Read the model definition and answer for the solid it produces. Units are mm, in the model's axes. Face numbers are marked on the shaded views. A direction names the side the tool comes from. Give positions to 0.01 mm unless a question says otherwise; leave off trailing zeros. Order: outer loops, then holes, each group sorted by start corner. A loop starts at its lowest first (then second) coordinate and runs counter-clockwise, first axis right, second up. Notation, with made-up numbers: M 85.25,66 L 132.25,66 A7 ccw 132.25,73 Z; hole C 72.5,-2.75 d4. An arc over 180 degrees is marked long. One line per item, written item: value. Start each with the question number.
Autodesk Inventor part; units mm, degrees
ref_plane "YZ Plane" through (0, 0, 0) normal (1, 0, 0) x (0, 1, 0)
ref_plane "XZ Plane" through (0, 0, 0) normal (0, 1, 0) x (-1, 0, 0)
ref_plane "XY Plane" through (0, 0, 0) normal (0, 0, 1) x (1, 0, 0)
sketch "スケッチ1" plane through (0, 0, 0) normal (0, 1, 0) x (-1, 0, 0)
  circle A0 centre (0, 0) radius 32.5
  dimension "d0" = 65
extrude "押し出し1" add sketch "スケッチ1" along normal blind 5.8
sketch "スケッチ2" plane through (0, 5.8, 0) normal (0, 1, 0) x (1, 0, 0)
  circle A0 centre (0, 0) radius 18
  dimension "d3" = 36
extrude "押し出し2" cut sketch "スケッチ2" against normal through all
sketch "スケッチ3" plane through (0, 0, 0) normal (0, -1, 0) x (1, 0, 0)
  circle A0 centre (0, 0) radius 25.15
  dimension "d6" = 50.3
extrude "押し出し3" cut sketch "スケッチ3" against normal blind 5.3
sketch "スケッチ4" plane through (0, 5.8, 0) normal (0, 1, 0) x (1, 0, 0)
  circle A0 centre (0, 0) radius 32.5
  circle A1 centre (0, 0) radius 25.65
  dimension "d9" = 51.3
extrude "押し出し4" cut sketch "スケッチ4" against normal blind 5.3
sketch "スケッチ5" plane through (0, 0.5, 0) normal (0, 1, 0) x (1, 0, 0)
  circle A0 centre (0, 29) radius 1.65
  circle A1 centre (-25.1147, -14.5) radius 1.65
  circle A2 centre (25.1147, -14.5) radius 1.65
  point P0 (0, 0)
  dimension "d12" = 3.3
  dimension "d13" = 29
  dimension "d16" = 360
extrude "押し出し5" cut sketch "スケッチ5" against normal through all
properties part number "clamp_for_bearing" material "ステンレス鋼"
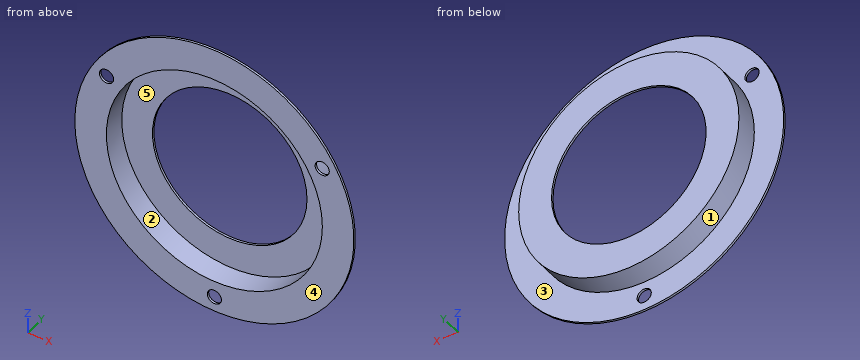
Q1. Find section C-C, the plane x = -17. Give the vertices of the cut face in (y, z), then the cut area to 3 significant figures.
Q2. Find section A-A, the plane x = 0. Give the vertices of the cut face in (y, z).
Q3. Determine the mould class of the marked faces 1, 2 and 3 for opening direction X: released by +X, released by -X, zero draft, split by the parting line, or undercut.
Q4. Consider probe 1 along X at (y, z) = (0.2, 14.5); probe 2 along X at (y, z) = (0.85, -0.5); probe 3 along X at (y, z) = (5.55, 0). Determine where each line is inside the solid, lowest interval first.
Q5. Find section B-B, the plane z = 0. Give the vertices of the cut face in (x, y).
Q6. A tool of negligible diameter and unlimited length cuts with its end or side. For the marked faces 4 and 5, from which of +Z, -Z, +X, -X, +Y, -Y can it reach the whole face along a straight path? Write none if from no direction.
Q7. Find section D-D, the plane z = 14.5. Give the vertices of the cut face in (x, y), then the cut area to 3 significant figures.
Q8. Each of these flat-tipped pins is pushed along its axis until it touches: pin 1 (4.5 mm diameter, centred on x = 25.11, z = 14.5, fed in from +Y); pin 2 (25 mm diameter, centred on x = -7, z = -5, fed in from -Y); pin 3 (1 mm diameter, centred on x = -13.5, y = 0.5, fed in from +Z). Where does it stop, or does it pass through?
Evaluation:
1. outline: M 0,-27.7 L 0.5,-27.7 L 0.5,-19.21 L 5.8,-19.21 L 5.8,-5.92 L 5.3,-5.92 L 5.3,-18.53 L 0,-18.53 Z; M 0,18.53 L 5.3,18.53 L 5.3,5.92 L 5.8,5.92 L 5.8,19.21 L 0.5,19.21 L 0.5,27.7 L 0,27.7 Z
1. area: 28.9 mm2
2. outline: M 0,-32.5 L 0.5,-32.5 L 0.5,-30.65 L 0,-30.65 Z; M 0,-27.35 L 0.5,-27.35 L 0.5,-25.65 L 5.8,-25.65 L 5.8,-18 L 5.3,-18 L 5.3,-25.15 L 0,-25.15 Z; M 0,25.15 L 5.3,25.15 L 5.3,18 L 5.8,18 L 5.8,25.65 L 0.5,25.65 L 0.5,32.5 L 0,32.5 Z
3. face 1: split by the parting line
3. face 2: undercut
3. face 3: zero draft
4. probe 1: -29.09 to -26.76, -23.46 to -20.55, 20.55 to 23.46, 26.76 to 29.09
4. probe 2: -25.65 to -25.15, 25.15 to 25.65
4. probe 3: -25.65 to -18, 18 to 25.65
5. outline: M -32.5,0 L -25.15,0 L -25.15,5.3 L -18,5.3 L -18,5.8 L -25.65,5.8 L -25.65,0.5 L -32.5,0.5 Z; M 18,5.3 L 25.15,5.3 L 25.15,0 L 32.5,0 L 32.5,0.5 L 25.65,0.5 L 25.65,5.8 L 18,5.8 Z
6. face 4: +Z, -Z, +X, -X, -Y
6. face 5: -Y
7. outline: M -29.09,0 L -26.76,0 L -26.76,0.5 L -29.09,0.5 Z; M -23.46,0 L -20.55,0 L -20.55,5.3 L -10.67,5.3 L -10.67,5.8 L -21.16,5.8 L -21.16,0.5 L -23.46,0.5 Z; M 10.67,5.3 L 20.55,5.3 L 20.55,0 L 23.46,0 L 23.46,0.5 L 21.16,0.5 L 21.16,5.8 L 10.67,5.8 Z; M 26.76,0 L 29.09,0 L 29.09,0.5 L 26.76,0.5 Z
7. area: 21.6 mm2
8. pin 1: y = 0.5
8. pin 2: y = 5.3
8. pin 3: z = 29.79
